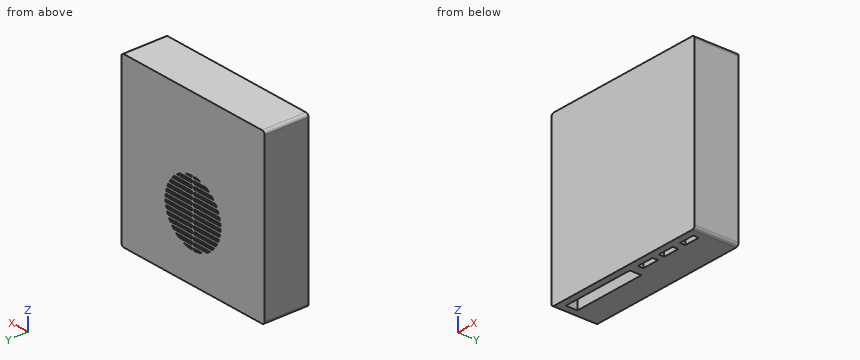
```python
from build123d import *

# Parameters (mm, degrees)
SKETCH_1_W          = 110
SKETCH_1_H          = 110
EXTRUDE_1_DEPTH     = 29
CUT_EXTRUDE_1_DEPTH = 7
SKETCH_3_W          = 53.883979218
SKETCH_3_H          = 56.07244117
CUT_EXTRUDE_3_DEPTH = 6
SKETCH_4_W          = 10.323301276
SKETCH_4_H          = 3.598949069
SKETCH_4_W_2        = 10.796847207
SKETCH_4_W_3        = 11.270393137
SKETCH_4_W_4        = 49.154067547
SKETCH_4_H_2        = 7.671444068
CUT_EXTRUDE_4_DEPTH = 10
FILLET_1_R          = 2


with BuildPart() as part:
    # 草图1 → 凸台-拉伸1 (new body)
    with BuildSketch(Plane(origin=(0, 0, 0), x_dir=(1, 0, 0), z_dir=(0, 1, 0))):
        Rectangle(SKETCH_1_W, SKETCH_1_H)
    extrude(amount=EXTRUDE_1_DEPTH)

    # 草图2 → 切除-拉伸1 (cut)
    with BuildSketch(Plane(origin=(0, 29, 0), x_dir=(1, 0, 0), z_dir=(0, 1, 0))):
        with BuildLine():
            Line((-0.751901528, 34.886318516), (-0.751901528, 33.59149031))
            Line((-0.751901528, 33.59149031), (-7.310776634, 33.59149031))
            ThreePointArc((-7.310776634, 33.59149031), (-4.082993976, 34.500559204), (-0.751901528, 34.886318516))
        make_face()
        with BuildLine():
            Line((-0.751901528, 31.99149031), (-0.751901528, 30.39149031))
            Line((-0.751901528, 30.39149031), (-13.029015886, 30.39149031))
            ThreePointArc((-13.029015886, 30.39149031), (-11.883781834, 31.230990299), (-10.684631719, 31.99149031))
            Line((-10.684631719, 31.99149031), (-0.751901528, 31.99149031))
        make_face()
        with BuildLine():
            Line((0.751901528, 34.886318516), (0.751901528, 33.59149031))
            Line((0.751901528, 33.59149031), (7.310776634, 33.59149031))
            ThreePointArc((7.310776634, 33.59149031), (4.082993976, 34.500559204), (0.751901528, 34.886318516))
        make_face()
        with BuildLine():
            Line((-14.840119775, 28.79149031), (-0.751901528, 28.79149031))
            Line((-0.751901528, 28.79149031), (-0.751901528, 27.19149031))
            Line((-0.751901528, 27.19149031), (-16.296719146, 27.19149031))
            ThreePointArc((-16.296719146, 27.19149031), (-15.588960341, 28.010190206), (-14.840119775, 28.79149031))
        make_face()
        with BuildLine():
            Line((-17.487622906, 25.59149031), (-0.751901528, 25.59149031))
            Line((-0.751901528, 25.59149031), (-0.751901528, 23.99149031))
            Line((-0.751901528, 23.99149031), (-18.464313009, 23.99149031))
            ThreePointArc((-18.464313009, 23.99149031), (-17.993760697, 24.802351555), (-17.487622906, 25.59149031))
        make_face()
        with BuildLine():
            Line((-19.259406919, 22.39149031), (-0.751901528, 22.39149031))
            Line((-0.751901528, 22.39149031), (-0.751901528, 20.79149031))
            Line((-0.751901528, 20.79149031), (-19.894689112, 20.79149031))
            ThreePointArc((-19.894689112, 20.79149031), (-19.593386869, 21.597977674), (-19.259406919, 22.39149031))
        make_face()
        with BuildLine():
            Line((-20.385106201, 19.19149031), (-0.751901528, 19.19149031))
            Line((-0.751901528, 19.19149031), (-0.751901528, 17.59149031))
            Line((-0.751901528, 17.59149031), (-20.740936691, 17.59149031))
            ThreePointArc((-20.740936691, 17.59149031), (-20.578577477, 18.394949879), (-20.385106201, 19.19149031))
        make_face()
        with BuildLine():
            Line((-20.969033235, 15.99149031), (-0.751901528, 15.99149031))
            Line((-0.751901528, 15.99149031), (-0.751901528, 14.39149031))
            Line((-0.751901528, 14.39149031), (-21.073543954, 14.39149031))
            ThreePointArc((-21.073543954, 14.39149031), (-21.03650575, 15.192484283), (-20.969033235, 15.99149031))
        make_face()
        with BuildLine():
            Line((-21.056309144, 12.79149031), (-0.751901528, 12.79149031))
            Line((-0.751901528, 12.79149031), (-0.751901528, 11.19149031))
            Line((-0.751901528, 11.19149031), (-20.917027866, 11.19149031))
            ThreePointArc((-20.917027866, 11.19149031), (-21.001910745, 11.990163461), (-21.056309144, 12.79149031))
        make_face()
        with BuildLine():
            Line((-20.653231097, 9.59149031), (-0.751901528, 9.59149031))
            Line((-0.751901528, 9.59149031), (-0.751901528, 7.99149031))
            Line((-0.751901528, 7.99149031), (-20.260055644, 7.99149031))
            ThreePointArc((-20.260055644, 7.99149031), (-20.472280234, 8.787647791), (-20.653231097, 9.59149031))
        make_face()
        with BuildLine():
            Line((-19.729768237, 6.39149031), (-0.751901528, 6.39149031))
            Line((-0.751901528, 6.39149031), (-0.751901528, 4.79149031))
            Line((-0.751901528, 4.79149031), (-19.050922672, 4.79149031))
            ThreePointArc((-19.050922672, 4.79149031), (-19.406841496, 5.584491395), (-19.729768237, 6.39149031))
        make_face()
        with BuildLine():
            Line((-18.206909531, 3.19149031), (-0.751901528, 3.19149031))
            Line((-0.751901528, 3.19149031), (-0.751901528, 1.59149031))
            Line((-0.751901528, 1.59149031), (-17.173393801, 1.59149031))
            ThreePointArc((-17.173393801, 1.59149031), (-17.708231587, 2.379811633), (-18.206909531, 3.19149031))
        make_face()
        with BuildLine():
            Line((-15.91349599, -0.00850969), (-0.751901528, -0.00850969))
            Line((-0.751901528, -0.00850969), (-0.751901528, -1.60850969))
            Line((-0.751901528, -1.60850969), (-14.367785306, -1.60850969))
            ThreePointArc((-14.367785306, -1.60850969), (-15.161761086, -0.828913494), (-15.91349599, -0.00850969))
        make_face()
        with BuildLine():
            Line((-12.430090691, -3.20850969), (-0.751901528, -3.20850969))
            Line((-0.751901528, -3.20850969), (-0.751901528, -4.80850969))
            Line((-0.751901528, -4.80850969), (-9.872236553, -4.80850969))
            ThreePointArc((-9.872236553, -4.80850969), (-11.17982335, -4.054326816), (-12.430090691, -3.20850969))
        make_face()
        with BuildLine():
            Line((-5.940955693, -6.40850969), (-0.751901528, -6.40850969))
            Line((-0.751901528, -6.40850969), (-0.751901528, -7.249525385))
            ThreePointArc((-0.751901528, -7.249525385), (-3.372745364, -6.991391514), (-5.940955693, -6.40850969))
        make_face()
        with BuildLine():
            Line((0.751901528, 31.99149031), (0.751901528, 30.39149031))
            Line((0.751901528, 30.39149031), (13.029015886, 30.39149031))
            ThreePointArc((13.029015886, 30.39149031), (11.883781834, 31.230990299), (10.684631719, 31.99149031))
            Line((10.684631719, 31.99149031), (0.751901528, 31.99149031))
        make_face()
        with BuildLine():
            Line((0.751901528, 28.79149031), (0.751901528, 27.19149031))
            Line((0.751901528, 27.19149031), (16.296719146, 27.19149031))
            ThreePointArc((16.296719146, 27.19149031), (15.588960341, 28.010190206), (14.840119775, 28.79149031))
            Line((14.840119775, 28.79149031), (0.751901528, 28.79149031))
        make_face()
        with BuildLine():
            Line((0.751901528, 25.59149031), (17.487622906, 25.59149031))
            ThreePointArc((17.487622906, 25.59149031), (17.993760697, 24.802351555), (18.464313009, 23.99149031))
            Line((18.464313009, 23.99149031), (0.751901528, 23.99149031))
            Line((0.751901528, 23.99149031), (0.751901528, 25.59149031))
        make_face()
        with BuildLine():
            Line((0.751901528, 22.39149031), (19.259406919, 22.39149031))
            ThreePointArc((19.259406919, 22.39149031), (19.593386869, 21.597977674), (19.894689112, 20.79149031))
            Line((19.894689112, 20.79149031), (0.751901528, 20.79149031))
            Line((0.751901528, 20.79149031), (0.751901528, 22.39149031))
        make_face()
        with BuildLine():
            Line((0.751901528, 19.19149031), (20.385106201, 19.19149031))
            ThreePointArc((20.385106201, 19.19149031), (20.578577477, 18.394949879), (20.740936691, 17.59149031))
            Line((20.740936691, 17.59149031), (0.751901528, 17.59149031))
            Line((0.751901528, 17.59149031), (0.751901528, 19.19149031))
        make_face()
        with BuildLine():
            Line((0.751901528, 15.99149031), (20.969033235, 15.99149031))
            ThreePointArc((20.969033235, 15.99149031), (21.03650575, 15.192484283), (21.073543954, 14.39149031))
            Line((21.073543954, 14.39149031), (0.751901528, 14.39149031))
            Line((0.751901528, 14.39149031), (0.751901528, 15.99149031))
        make_face()
        with BuildLine():
            Line((0.751901528, 12.79149031), (21.056309144, 12.79149031))
            ThreePointArc((21.056309144, 12.79149031), (21.001910745, 11.990163461), (20.917027866, 11.19149031))
            Line((20.917027866, 11.19149031), (0.751901528, 11.19149031))
            Line((0.751901528, 11.19149031), (0.751901528, 12.79149031))
        make_face()
        with BuildLine():
            Line((0.751901528, 9.59149031), (20.653231097, 9.59149031))
            ThreePointArc((20.653231097, 9.59149031), (20.472280234, 8.787647791), (20.260055644, 7.99149031))
            Line((20.260055644, 7.99149031), (0.751901528, 7.99149031))
            Line((0.751901528, 7.99149031), (0.751901528, 9.59149031))
        make_face()
        with BuildLine():
            Line((0.751901528, 6.39149031), (19.729768237, 6.39149031))
            ThreePointArc((19.729768237, 6.39149031), (19.406841496, 5.584491395), (19.050922672, 4.79149031))
            Line((19.050922672, 4.79149031), (0.751901528, 4.79149031))
            Line((0.751901528, 4.79149031), (0.751901528, 6.39149031))
        make_face()
        with BuildLine():
            Line((0.751901528, 3.19149031), (18.206909531, 3.19149031))
            ThreePointArc((18.206909531, 3.19149031), (17.708231587, 2.379811633), (17.173393801, 1.59149031))
            Line((17.173393801, 1.59149031), (0.751901528, 1.59149031))
            Line((0.751901528, 1.59149031), (0.751901528, 3.19149031))
        make_face()
        with BuildLine():
            Line((0.751901528, -0.00850969), (15.91349599, -0.00850969))
            ThreePointArc((15.91349599, -0.00850969), (15.161761086, -0.828913494), (14.367785306, -1.60850969))
            Line((14.367785306, -1.60850969), (0.751901528, -1.60850969))
            Line((0.751901528, -1.60850969), (0.751901528, -0.00850969))
        make_face()
        with BuildLine():
            Line((0.751901528, -3.20850969), (12.430090691, -3.20850969))
            ThreePointArc((12.430090691, -3.20850969), (11.17982335, -4.054326816), (9.872236553, -4.80850969))
            Line((9.872236553, -4.80850969), (0.751901528, -4.80850969))
            Line((0.751901528, -4.80850969), (0.751901528, -3.20850969))
        make_face()
        with BuildLine():
            Line((0.751901528, -6.40850969), (5.940955693, -6.40850969))
            ThreePointArc((5.940955693, -6.40850969), (3.372745364, -6.991391514), (0.751901528, -7.249525385))
            Line((0.751901528, -7.249525385), (0.751901528, -6.40850969))
        make_face()
    extrude(amount=-CUT_EXTRUDE_1_DEPTH, mode=Mode.SUBTRACT)

    # 草图3 → 切除-拉伸3 (cut)
    with BuildSketch(Plane(origin=(0, 22, 0), x_dir=(1, 0, 0), z_dir=(0, 1, 0))):
        with Locations((-2.446069618, 15.99149031)):
            Rectangle(SKETCH_3_W, SKETCH_3_H)
    extrude(amount=CUT_EXTRUDE_3_DEPTH, mode=Mode.SUBTRACT)

    # 草图4 → 切除-拉伸4 (cut)
    with BuildSketch(Plane(origin=(0, 0, -55), x_dir=(-1, 0, 0), z_dir=(0, 0, -1))):
        with Locations((-43.710945988, 6.201665953)):
            Rectangle(SKETCH_4_W, SKETCH_4_H)
        with Locations((-27.657738957, 6.201665953)):
            Rectangle(SKETCH_4_W_2, SKETCH_4_H)
        with Locations((-11.888659484, 6.201665953)):
            Rectangle(SKETCH_4_W_3, SKETCH_4_H)
        with Locations((24.47966795, 8.237913452)):
            Rectangle(SKETCH_4_W_4, SKETCH_4_H_2)
    extrude(amount=-CUT_EXTRUDE_4_DEPTH, mode=Mode.SUBTRACT)

    # 圆角1
    fillet_1_edges = [part.edges().sort_by_distance(p)[0] for p in [
        (-55, 14.5, -55),
        (55, 14.5, -55),
        (55, 14.5, 55),
        (-55, 14.5, 55),
    ]]
    fillet(fillet_1_edges, radius=FILLET_1_R)


solid = part.part
```
Geometry check sheet. Reference: the model listing, model coordinates, mm. Round coordinates to 2 decimals unless told otherwise and drop trailing zeros. Order: outer loops, then holes, each group sorted by start corner. A loop starts at its lowest first (then second) coordinate and runs counter-clockwise, first axis right, second up. Notation, with made-up numbers: (11.5, -27.5) - (65.5, -27.5) arc R21 ccw to (65.5, -2.5) - close; hole circle Ø5 at (74.5, 42). An arc over 180 degrees is marked (long way). Use a Markdown table: item, result. Add a question column.
1) Section check B-B (y = 5.75). Record the cut outline in (x, z).
2) Section check A-A (y = 25.75). Record the cut outline in (x, z).
3) Section check C-C (x = 3). Count the separate pieces of the cut face and the enclosed holes in it, then the cut area to 3 significant figures.
4) Thickness scan on line 1 along Y through (x, z) = (4, -30); line 2 along Z through (x, y) = (9, 27.5); line 3 along Z through (x, y) = (-15, 10.75). Record the ranges inside material, lowest first.
Established:
| question | item | result |
|---|---|---|
| 1 | outline | (-55, -53) arc R2 ccw to (-53, -55) - (-49.06, -55) - (-49.06, -45) - (0.1, -45) - (0.1, -55) - (6.25, -55) - (6.25, -45) - (17.52, -45) - (17.52, -55) - (22.26, -55) - (22.26, -45) - (33.06, -45) - (33.06, -55) - (38.55, -55) - (38.55, -45) - (48.87, -45) - (48.87, -55) - (53, -55) arc R2 ccw to (55, -53) - (55, 53) arc R2 ccw to (53, 55) - (-53, 55) arc R2 ccw to (-55, 53) - close |
| 2 | outline | (-55, -53) arc R2 ccw to (-53, -55) - (53, -55) arc R2 ccw to (55, -53) - (55, 53) arc R2 ccw to (53, 55) - (-53, 55) arc R2 ccw to (-55, 53) - close; hole (-29.39, -44.03) - (24.5, -44.03) - (24.5, 12.04) - (-29.39, 12.04) - close |
| 3 | separate pieces | 14 |
| 3 | enclosed holes | 0 |
| 3 | area | 2,830 mm2 |
| 4 | line 1 | 0 to 22, 28 to 29 |
| 4 | line 2 | -55 to -44.03, 12.04 to 55 |
| 4 | line 3 | -45 to 55 |
